The model under review builds one solid part; all positions refer to its coordinate system, in mm. A direction names the side the tool comes from. Give positions to 0.01 mm unless a question says otherwise; leave off trailing zeros. Loops run counter-clockwise (first coordinate to the right, second up) from the corner with the lowest first, then second, coordinate; pieces in that order, holes last. Notation, with made-up numbers: (58.5, -37) - (81.5, -37) arc R13 cw to (81.5, -23) - close; hole circle Ø4 at (31.25, 4). An arc over 180 degrees is marked (long way). Answer as a JSON object with one key per item and string values.
from build123d import *

# Parameters (mm, degrees)
F0_W     = 300
F0_H     = 300
F0_W_2   = 280
F0_H_2   = 135
F1_DEPTH = 300
F2_R     = 20
F3_R     = 25


with BuildPart() as f1:
    # F0 (on Front) → F1 (new body)
    with BuildSketch(Plane.XZ):
        with Locations((150, 150)):
            Rectangle(F0_W, F0_H)
        with Locations((150, 77.5)):
            Rectangle(F0_W_2, F0_H_2, mode=Mode.SUBTRACT)
        with Locations((150, 222.5)):
            Rectangle(F0_W_2, F0_H_2, mode=Mode.SUBTRACT)
    extrude(amount=F1_DEPTH)

    # F2
    f2_edges = [f1.edges().sort_by_distance(p)[0] for p in [
        (10, -150, 290),
        (10, -150, 145),
        (290, -150, 290),
        (290, -150, 145),
        (10, -150, 155),
        (290, -150, 155),
        (290, -150, 10),
        (10, -150, 10),
    ]]
    fillet(f2_edges, radius=F2_R)

    # F3
    f3_edges = [f1.edges().sort_by_distance(p)[0] for p in [
        (0, -150, 300),
        (300, -150, 300),
        (300, -150, 0),
        (0, -150, 0),
    ]]
    fillet(f3_edges, radius=F3_R)


solid = f1.part
Q1. The part is to be moulded in two halves that separate along X. For faces 3 (the face through (0, -148, 148)), 4 (the face through (148, -148, 155)), 5 (the face through (300, -148, 148)), say which applies: +X half, -X half, draft (parallel to the pull), parting line (faces both ways), or undercut.
Results:
{"face 3": "-X half", "face 4": "undercut", "face 5": "+X half"}
Q2. For faces 1 (the face through (292.482, -152.1, 292.871)), 2 (the face through (148, -148, 10)), list the 3-axis set-ups (+Z, -Z, +X, -X, +Y, -Y) from which the entire face can be reached by the end or side of a thin tool; tool diameter is ignored.
Results:
{"face 1": "+Z, +X, +Y, -Y", "face 2": "+Y, -Y"}
Q3. Consider section C-C, the plane x = 230. State the section outline as (y, z) points.
Results:
{"outline": "(-300, 0) - (0, 0) - (0, 10) - (-300, 10) - close; (-300, 145) - (0, 145) - (0, 155) - (-300, 155) - close; (-300, 290) - (0, 290) - (0, 300) - (-300, 300) - close"}
Q4. To check wall thickness, follow probe 1 along Z at (x, y) = (102.5, -79.5); probe 2 along X at (y, z) = (-199.5, 216); probe 3 along Z at (x, y) = (274, -118). State the ranges of each line that lie inside material, in increasing order. Write a range as [from, to].
Results:
{"probe 1": "z = [0, 10], [145, 155], [290, 300]", "probe 2": "x = [0, 10], [290, 300]", "probe 3": "z = [0, 10.4], [144.6, 155.4], [289.6, 300]"}
Q5. Consider section D-D, the plane x = 19.5. State the section outline as (y, z) points, plus the area to 3 significant figures.
Results:
{"outline": "(-300, 0.61) - (0, 0.61) - (0, 12.98) - (-300, 12.98) - close; (-300, 142.02) - (0, 142.02) - (0, 157.98) - (-300, 157.98) - close; (-300, 287.02) - (0, 287.02) - (0, 299.39) - (-300, 299.39) - close", "area": "12,200 mm^2"}
Q6. Consider section B-B, the plane y = -240. State the section outline as (x, z) points, plus the area to 3 significant figures.
Results:
{"outline": "(0, 25) arc R25 ccw to (25, 0) - (275, 0) arc R25 ccw to (300, 25) - (300, 275) arc R25 ccw to (275, 300) - (25, 300) arc R25 ccw to (0, 275) - close; hole (10, 30) arc R20 ccw to (30, 10) - (270, 10) arc R20 ccw to (290, 30) - (290, 125) arc R20 ccw to (270, 145) - (30, 145) arc R20 ccw to (10, 125) - close; hole (10, 175) arc R20 ccw to (30, 155) - (270, 155) arc R20 ccw to (290, 175) - (290, 270) arc R20 ccw to (270, 290) - (30, 290) arc R20 ccw to (10, 270) - close", "area": "14,600 mm^2"}
Q7. Consider section A-A, the plane z = 36.5. State the section outline as (x, y) points.
Results:
{"outline": "(0, -300) - (10, -300) - (10, 0) - (0, 0) - close; (290, -300) - (300, -300) - (300, 0) - (290, 0) - close"}
